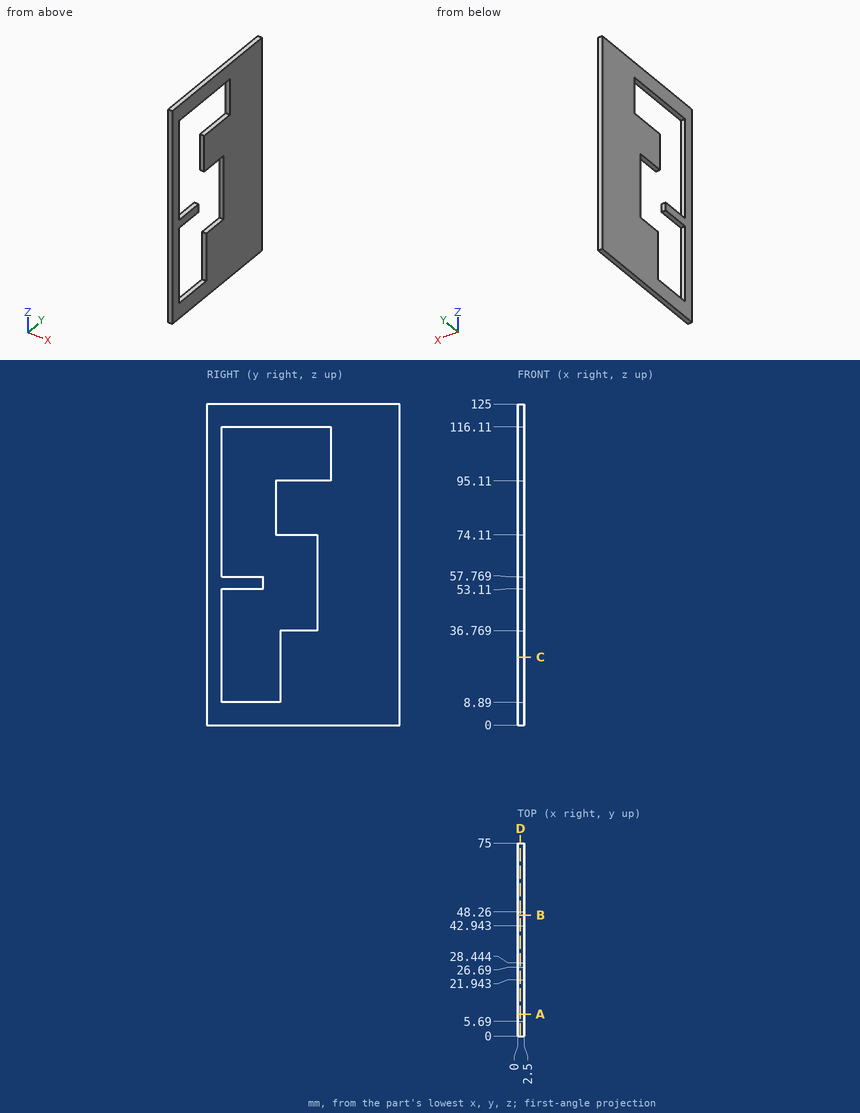
Could you check a few things on this drawing? It's one solid part, dimensions in mm from its lowest x, y, z. Give positions to 0.01 mm unless a question says otherwise; leave off trailing zeros. Write each loop counter-clockwise with the first axis right and the second up, starting at its lowest first coordinate (ties: lowest second). Pieces come first, ordered by that corner, then holes.
(1) Imagine slicing it at D-D, the plane x = 1.1. Write out the boundary of the cut face in (y, z) (1 decimal).
Output values:
outline: (0, 0) - (75, 0) - (75, 125) - (0, 125) - close; hole (5.7, 8.9) - (28.4, 8.9) - (28.4, 36.8) - (42.9, 36.8) - (42.9, 74.1) - (26.7, 74.1) - (26.7, 95.1) - (48.3, 95.1) - (48.3, 116.1) - (5.7, 116.1) - (5.7, 57.8) - (21.9, 57.8) - (21.9, 53.1) - (5.7, 53.1) - close
(2) Will this pin go through, and if not, where does the flat tip stop? pin 1 (0.8 mm diameter, centred on x = 1, y = 16.5, fed in from -Z).
Output values:
pin 1: stops at z = 0
(3) Imagine slicing it at B-B, the plane y = 47. Write out the boundary of the cut face in (x, z).
Output values:
outline: (0, 0) - (2.5, 0) - (2.5, 95.11) - (0, 95.11) - close; (0, 116.11) - (2.5, 116.11) - (2.5, 125) - (0, 125) - close
(4) Imagine slicing it at A-A, the plane y = 8.5. Write out the boundary of the cut face in (x, z).
Output values:
outline: (0, 0) - (2.5, 0) - (2.5, 8.89) - (0, 8.89) - close; (0, 53.11) - (2.5, 53.11) - (2.5, 57.77) - (0, 57.77) - close; (0, 116.11) - (2.5, 116.11) - (2.5, 125) - (0, 125) - close
(5) If I drill on L1, parallel to Z at x = 0.45, y = 30.5; L2, parallel to Z at x = 1.4, y = 21; L3, parallel to Y at x = 0.5, z = 15 (1 decimal), over which ranges is the centre line in solid material (lowest first)?
Output values:
L1: z = 0 to 36.77, 74.11 to 95.11, 116.11 to 125
L2: z = 0 to 8.89, 53.11 to 57.77, 116.11 to 125
L3: y = 0 to 5.7, 28.4 to 75
(6) Imagine slicing it at C-C, the plane z = 26.5. Write out the boundary of the cut face in (x, y) (1 decimal), and give its area (3 significant figures).
Output values:
outline: (0, 0) - (2.5, 0) - (2.5, 5.7) - (0, 5.7) - close; (0, 28.4) - (2.5, 28.4) - (2.5, 75) - (0, 75) - close
area: 131 mm2
